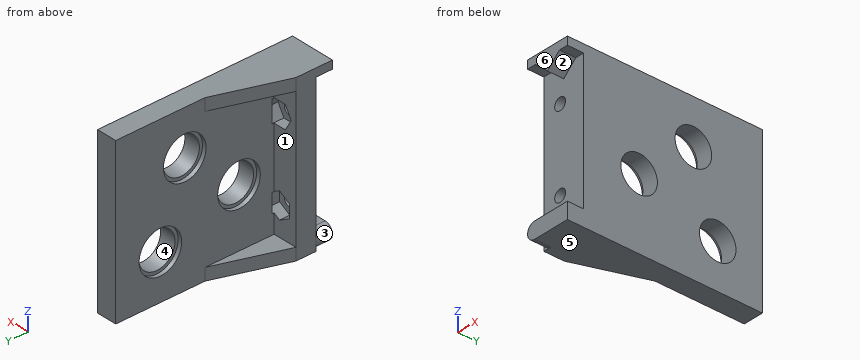
```python
from build123d import *

# Parameters (mm, degrees)
SKETCH_1_W               = 40
SKETCH_1_H               = 44
SKETCH_1_R               = 4.5
EXTRUDE_1_DEPTH          = 5
SKETCH_2_R               = 5.25
CUT_EXTRUDE_1_DEPTH      = 1
SKETCH_3_W               = 40
SKETCH_3_H               = 5
EXTRUDE_2_DEPTH          = 6
EXTRUDE_3_DEPTH          = 4
SKETCH_5_R               = 1.5
CUT_EXTRUDE_2_DEPTH      = 5
CUT_EXTRUDE_3_DEPTH      = 0.5
CUT_EXTRUDE_3_DEPTH_BACK = 2.5
EXTRUDE_4_DEPTH          = 3
EXTRUDE_5_DEPTH          = 3


with BuildPart() as part:
    # 草图1 → 凸台-拉伸1 (new body)
    with BuildSketch(Plane(origin=(0, 0, 0), x_dir=(0, 0, -1), z_dir=(1, 0, 0))):
        with Locations((9, -5)):
            Rectangle(SKETCH_1_W, SKETCH_1_H)
        Circle(SKETCH_1_R, mode=Mode.SUBTRACT)
        with Locations((18, 6)):
            Circle(SKETCH_1_R, mode=Mode.SUBTRACT)
        with Locations((11.543885882, -13.351449313)):
            Circle(SKETCH_1_R, mode=Mode.SUBTRACT)
    extrude(amount=EXTRUDE_1_DEPTH)

    # 草图2 → 切除-拉伸1 (cut)
    with BuildSketch(Plane.ZY):
        with Locations((-18, 6)):
            Circle(SKETCH_2_R)
        Circle(SKETCH_2_R)
        with Locations((-11.543885882, -13.351449313)):
            Circle(SKETCH_2_R)
    extrude(amount=-CUT_EXTRUDE_1_DEPTH, mode=Mode.SUBTRACT)

    # 草图3 → 凸台-拉伸2 (add)
    with BuildSketch(Plane.ZY):
        with Locations((-9, -24.5)):
            Rectangle(SKETCH_3_W, SKETCH_3_H)
    extrude(amount=EXTRUDE_2_DEPTH)

    # 草图4 → 凸台-拉伸3 (add)
    with BuildSketch(Plane.XZ.offset(27)):
        Polygon((5, 11), (-6, 11), (-6, 9), (-3.8, 9), (-0.5, 6), (2.8, 9), (5, 9), align=None)
        with BuildLine():
            Line((5, -29), (-4, -29))
            ThreePointArc((-4, -29), (-6, -27), (-4, -25))
            Line((-4, -25), (5, -25))
            Line((5, -25), (5, -29))
        make_face()
    extrude(amount=EXTRUDE_3_DEPTH)

    # 草图5 → 切除-拉伸2 (cut)
    with BuildSketch(Plane.XZ.offset(27)):
        with Locations((-1.5, -19)):
            Circle(SKETCH_5_R)
        with Locations((-1.5, 1)):
            Circle(SKETCH_5_R)
    extrude(amount=-CUT_EXTRUDE_2_DEPTH, mode=Mode.SUBTRACT)

    # 草图6 → 切除-拉伸3 (cut, two sides)
    with BuildSketch(Plane(origin=(0, -22, 0), x_dir=(1, 0, 0), z_dir=(0, 1, 0))) as cut_extrude_3_sk:
        Polygon((-1.5, 15.795706006), (1.275, 17.397853003), (1.275, 20.602146997), (-1.5, 22.204293994), (-4.275, 20.602146997), (-4.275, 17.397853003), align=None)
        Polygon((-4.704293994, -1), (-3.102146997, -3.775), (0.102146997, -3.775), (1.704293994, -1), (0.102146997, 1.775), (-3.102146997, 1.775), align=None)
    extrude(amount=CUT_EXTRUDE_3_DEPTH, mode=Mode.SUBTRACT)
    extrude(cut_extrude_3_sk.sketch, amount=-CUT_EXTRUDE_3_DEPTH_BACK, mode=Mode.SUBTRACT)

    # 草图7 → 凸台-拉伸4 (add)
    with BuildSketch(Plane.XY.offset(11)):
        Polygon((0, -22), (-6, -22), (0, -5), align=None)
    extrude(amount=-EXTRUDE_4_DEPTH)

    # 草图8 → 凸台-拉伸5 (add)
    with BuildSketch(Plane(origin=(0, 0, -29), x_dir=(-1, 0, 0), z_dir=(0, 0, -1))):
        Polygon((0, -22), (6, -22), (0, -5), align=None)
    extrude(amount=-EXTRUDE_5_DEPTH)


solid = part.part
```
Geometry check sheet. Reference: the model listing, model coordinates, mm. Face numbers are marked on the shaded views. A direction names the side the tool comes from. Round coordinates to 2 decimals unless told otherwise and drop trailing zeros. Loops run counter-clockwise (first coordinate to the right, second up) from the corner with the lowest first, then second, coordinate; pieces in that order, holes last. Notation, with made-up numbers: (12.5, -16) - (24.5, -16) arc R14 cw to (24.5, -6) - close; hole circle Ø7 at (26.25, 49.25). An arc over 180 degrees is marked (long way). Use a Markdown table: item, result.
Q1. Cross-section at D-D on z = -2.5. Record the cut outline in (x, y).
Solutions:
| item | result |
|---|---|
| outline | (-6, -27) - (5, -27) - (5, -3.74) - (1, -3.74) - (1, -4.62) - (0, -4.62) - (0, -22) - (-6, -22) - close; (0, 4.62) - (1, 4.62) - (1, 3.74) - (5, 3.74) - (5, 17) - (0, 17) - close |
Q2. Go/stop test with flat-tipped pins: P1, Ø6, axis at y = -14, z = -12, coming from the -X side; P2, Ø1.5, axis at y = -8, z = -2.5, coming from the -X side; P3, Ø0.9, axis at x = 1.5, z = 2, coming from the -Y side; P4, Ø1.8, axis at x = -5, y = -30, coming from the -Z side. Record where each tip stops, or that it passes through.
Solutions:
| item | result |
|---|---|
| P1 | passes through |
| P2 | stops at x = 0 |
| P3 | stops at y = -27 |
| P4 | stops at z = -29 |
Q3. Cross-section at B-B on z = -19. Record the cut outline in (x, y) (3 decimals), plus the area to 3 significant figures.
Solutions:
| item | result |
|---|---|
| outline | (-6, -27) - (-3, -27) - (-3, -24.5) - (-4.275, -24.5) - (-4.275, -22) - (-6, -22) - close; (0, -27) - (5, -27) - (5, 1.613) - (1, 1.613) - (1, 0.846) - (0, 0.846) - (0, -21.5) - (1.275, -21.5) - (1.275, -24.5) - (0, -24.5) - close; (0, 11.154) - (1, 11.154) - (1, 10.387) - (5, 10.387) - (5, 17) - (0, 17) - close |
| area | 183 mm2 |
Q4. Access from +Z, -Z, +X, -X, +Y, -Y to the whole of each face (thin tool, end or side, straight path). Record for the marked faces 1, 2 and 3.
Solutions:
| item | result |
|---|---|
| face 1 | -X, +Y |
| face 2 | +X, -Y |
| face 3 | -X, -Y |
Q5. Material ranges on line 1 (Y direction, x = 0.3, z = 0); line 2 (Z direction, x = -1.5, y = -25); line 3 (Y direction, x = 0.5, z = -16), recorded low to high.
Solutions:
| item | result |
|---|---|
| line 1 | y = -27 to -24.5, -21.5 to -5.25, 5.25 to 17 |
| line 2 | z = -29 to -20.5, -17.5 to -0.5, 2.5 to 11 |
| line 3 | y = -27 to -16.13, -10.58 to 1.15, 10.85 to 17 |
Q6. Cross-section at A-A on y = 6. Record the cut outline in (x, z), plus the area to 4 significant figures.
Solutions:
| item | result |
|---|---|
| outline | (0, -29) - (5, -29) - (5, -22.5) - (1, -22.5) - (1, -23.25) - (0, -23.25) - close; (0, -12.75) - (1, -12.75) - (1, -13.5) - (5, -13.5) - (5, 11) - (0, 11) - close |
| area | 153.5 mm2 |
Q7. Cross-section at C-C on z = -11.5. Record the cut outline in (x, y).
Solutions:
| item | result |
|---|---|
| outline | (-6, -27) - (5, -27) - (5, -17.85) - (1, -17.85) - (1, -18.6) - (0, -18.6) - (0, -22) - (-6, -22) - close; (0, -8.1) - (1, -8.1) - (1, -8.85) - (5, -8.85) - (5, 17) - (0, 17) - close |
Q8. Draft check along Z on the marked faces 4, 5 and 6. Enter one of: released by +Z, released by -Z, zero draft, split by the parting line, or undercut.
Solutions:
| item | result |
|---|---|
| face 4 | undercut |
| face 5 | released by -Z |
| face 6 | zero draft |
